Could you check a few things on this model? Use its own coordinates, in mm. Face numbers are marked on the shaded views. Give positions to 0.01 mm unless a question says otherwise; leave off trailing zeros. Write each loop counter-clockwise with the first axis right and the second up, starting at its lowest first coordinate (ties: lowest second). Pieces come first, ordered by that corner, then holes. Notation, with made-up numbers: (33.5, 75) - (88.5, 75) arc R24 ccw to (88.5, 101) - close; hole circle Ø1 at (27.5, -37). An arc over 180 degrees is marked (long way). Answer as CSV lines item,"result". Start each with the question number.
Q1. Imagine slicing it at C-C on z = 34. List the corners of the cut face in (x, y) for me, and give its area (3 significant figures).
Q2. Imagine slicing it at A-A on x = 0. List the corners of the cut face in (y, z) for me.
Q3. We'd pull the mould along X, two halves only. Please class the marked faces 1, 2 and 3: pulls with the +X half, pulls with the -X half, needs draft (parallel to the pull), parting line crosses it, or undercut.
Q4. If I drill on line 1 along Z through (x, y) = (0, 258); line 2 along X through (y, z) = (160, -0.5); line 3 along Y through (x, z) = (-32, 0), over which ranges is the centre line in solid material (lowest first)?
Q5. Imagine slicing it at D-D on y = 89. State how many separate pieces and enclosed holes the cut face has, and give its area (3 significant figures).
Q6. Will these pins go through, and if not, where does the flat tip stop? pin 1 Ø12 at (y, z) = (23.5, -20.5) entering from +X; pin 2 Ø5 at (x, y) = (-32, 140) entering from -Z; pin 3 Ø1 at (y, z) = (239, 28) entering from +X.
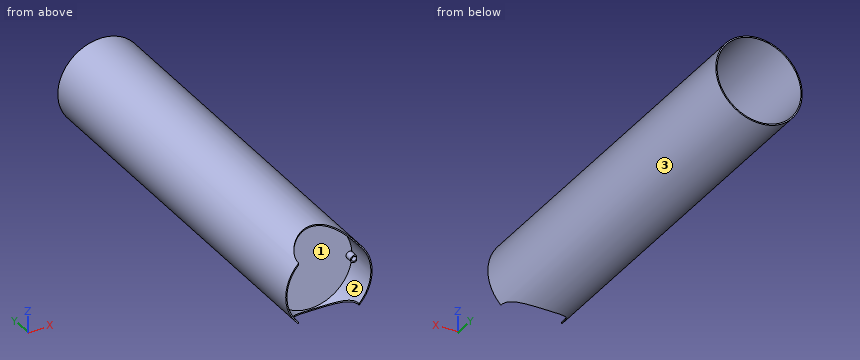
```python
from build123d import *

# Parameters (mm, degrees)
SKETCH1_R                        = 57.15
SKETCH1_R_2                      = 55.5625
OEM_DEPTH                        = 457.2
OEM_DEPTH_BACK                   = 152.4
ENSR_BASEPLATE_CUTOUT_DEPTH      = 58.15
ENSR_BASEPLATE_CUTOUT_DEPTH_BACK = 58.15
SKETCH6_W                        = 114.3
SKETCH6_H                        = 100
TOO_LONG_DEPTH                   = 58.1500001
TOO_LONG_DEPTH_BACK              = 58.1500001
SKETCH7_R                        = 4.7625
SKETCH7_R_2                      = 3.175
CONDUIT_DEPTH                    = 300
CONDUIT_DEPTH_BACK               = 10
SKETCH3_R                        = 57.15
SKETCH3_R_2                      = 3.175
FLOOR_2_DEPTH                    = 1.5875


with BuildPart() as part:
    # Sketch1 → OEM (new body, two sides)
    with BuildSketch(Plane(origin=(0, 0, 0), x_dir=(1, 0, 0), z_dir=(0, 1, 0))) as oem_sk:
        Circle(SKETCH1_R)
        Circle(SKETCH1_R_2, mode=Mode.SUBTRACT)
    extrude(amount=OEM_DEPTH)
    extrude(oem_sk.sketch, amount=-OEM_DEPTH_BACK)

    # Sketch5 → eNSR baseplate cutout (cut, two sides)
    with BuildSketch(Plane.XY) as ensr_baseplate_cutout_sk:
        with BuildLine():
            Line((40, -1396.985408143), (40, -152.4))
            ThreePointArc((40, -152.4), (0, -112.4), (-40, -152.4))
            Line((-40, -152.4), (-40, -1396.985408143))
            Line((-40, -1396.985408143), (-40, -3886.156224429))
            Line((-40, -3886.156224429), (40, -3886.156224429))
            Line((40, -3886.156224429), (40, -1396.985408143))
        make_face()
    extrude(amount=ENSR_BASEPLATE_CUTOUT_DEPTH, mode=Mode.SUBTRACT)
    extrude(ensr_baseplate_cutout_sk.sketch, amount=-ENSR_BASEPLATE_CUTOUT_DEPTH_BACK, mode=Mode.SUBTRACT)

    # Sketch6 → too long (cut, two sides)
    with BuildSketch(Plane.XY) as too_long_sk:
        with Locations((0, 407.2)):
            Rectangle(SKETCH6_W, SKETCH6_H)
    extrude(amount=TOO_LONG_DEPTH, mode=Mode.SUBTRACT)
    extrude(too_long_sk.sketch, amount=-TOO_LONG_DEPTH_BACK, mode=Mode.SUBTRACT)

    # Sketch7 → conduit (add, two sides)
    with BuildSketch(Plane(origin=(0, -110, 0), x_dir=(1, 0, 0), z_dir=(0, 1, 0))) as conduit_sk:
        with Locations((52.3875, 0)):
            Circle(SKETCH7_R)
        with Locations((52.3875, 0)):
            Circle(SKETCH7_R_2, mode=Mode.SUBTRACT)
    extrude(amount=CONDUIT_DEPTH)
    extrude(conduit_sk.sketch, amount=-CONDUIT_DEPTH_BACK)

    # Sketch3 → floor 2 (add)
    with BuildSketch(Plane(origin=(0, -110, 0), x_dir=(1, 0, 0), z_dir=(0, 1, 0))):
        Circle(SKETCH3_R)
        with Locations((52.3875, 0)):
            Circle(SKETCH3_R_2, mode=Mode.SUBTRACT)
    extrude(amount=FLOOR_2_DEPTH)


solid = part.part
```
Conclusion:
1,outline,"(-45.94, -152.4) - (-43.95, -152.4) - (-43.95, -110) - (43.95, -110) - (43.95, -152.4) - (45.94, -152.4) - (45.94, 357.2) - (43.95, 357.2) - (43.95, -108.41) - (-43.95, -108.41) - (-43.95, 357.2) - (-45.94, 357.2) - close"
1,area,"2,170 mm^2"
2,outline,"(-112.4, -57.15) - (357.2, -57.15) - (357.2, -55.56) - (-108.41, -55.56) - (-108.41, 55.56) - (357.2, 55.56) - (357.2, 57.15) - (-112.4, 57.15) - (-112.4, 55.56) - (-110, 55.56) - (-110, -55.56) - (-112.4, -55.56) - close"
3,face 1,"undercut"
3,face 2,"undercut"
3,face 3,"parting line crosses it"
4,line 1,"-57.15 to -55.56, 55.56 to 57.15"
4,line 2,"-57.15 to -55.56, 47.65 to 49.25, 55.52 to 57.15"
4,line 3,"-110 to -108.41"
5,separate pieces,"1"
5,enclosed holes,"2"
5,area,"594 mm^2"
6,pin 1,"x = 55.28"
6,pin 2,"z = -48.95"
6,pin 3,"x = 50.1"
